```python
from build123d import *

# Parameters (mm, degrees)
EXTRUDE_1_DEPTH              = 3
HOLE_WIZARD_M3_1_D           = 3.4
HOLE_WIZARD_M3_1_DEPTH       = 15
HOLE_WIZARD_M3_1_CSINK_D     = 6.3
HOLE_WIZARD_M3_1_CSINK_ANGLE = 90
HOLE_WIZARD_M3_1_TIP         = 1.021463052


with BuildPart() as part:
    # 草圖1 → 填料-伸長1 (new body)
    with BuildSketch(Plane.XY):
        Polygon((-57.5, -55), (57.5, -55), (57.5, 55), (47.5, 55), (47.5, 95), (-47.5, 95), (-47.5, 55), (-57.5, 55), align=None)
    extrude(amount=EXTRUDE_1_DEPTH)

    # M3 錐坑平頭螺釘的錐孔1
    with Locations(Plane.XY.offset(3)):
        with Locations((-52.5, -50), (-42.5, 90), (-42.5, 50), (42.5, 90), (42.5, 50), (52.5, -50)):
            CounterSinkHole(HOLE_WIZARD_M3_1_D / 2, HOLE_WIZARD_M3_1_CSINK_D / 2, depth=HOLE_WIZARD_M3_1_DEPTH, counter_sink_angle=HOLE_WIZARD_M3_1_CSINK_ANGLE)
            with Locations((0, 0, -(HOLE_WIZARD_M3_1_DEPTH + HOLE_WIZARD_M3_1_TIP / 2))):  # 118° drill point
                Cone(0, HOLE_WIZARD_M3_1_D / 2, HOLE_WIZARD_M3_1_TIP, mode=Mode.SUBTRACT)


solid = part.part
```
Geometry check sheet. Reference: the model listing, model coordinates, mm. A direction names the side the tool comes from. Round coordinates to 2 decimals unless told otherwise and drop trailing zeros. Write each loop counter-clockwise with the first axis right and the second up, starting at its lowest first coordinate (ties: lowest second). Pieces come first, ordered by that corner, then holes. Notation, with made-up numbers: (88, 44) -> (97, 44) arc R30 ccw to (97, 76) -> close; hole circle Ø7 at (20.5, 8.25). An arc over 180 degrees is marked (long way). Put each result on its own line as item: value.
1) Cross-section at C-C, the plane z = 2.3. Enter the section's corners in (x, y).
Recorded:
outline: (-57.5, -55) -> (57.5, -55) -> (57.5, 55) -> (47.5, 55) -> (47.5, 95) -> (-47.5, 95) -> (-47.5, 55) -> (-57.5, 55) -> close; hole circle Ø4.9 at (-52.5, -50); hole circle Ø4.9 at (-42.5, 50); hole circle Ø4.9 at (-42.5, 90); hole circle Ø4.9 at (42.5, 50); hole circle Ø4.9 at (42.5, 90); hole circle Ø4.9 at (52.5, -50)
2) Thickness scan on probe 1 along Y at (x, z) = (-42.5, 0.65); probe 2 along X at (y, z) = (-50, 0.95); probe 3 along Y at (x, z) = (52.5, 1). Record the ranges inside material, lowest first. Write a range as from..to.
Recorded:
probe 1: y = -55..48.3, 51.7..88.3, 91.7..95
probe 2: x = -57.5..-54.2, -50.8..50.8, 54.2..57.5
probe 3: y = -55..-51.7, -48.3..55
3) Cross-section at B-B, the plane x = -42.5. Enter the section's corners in (y, z).
Recorded:
outline: (-55, 0) -> (48.3, 0) -> (48.3, 1.55) -> (46.85, 3) -> (-55, 3) -> close; (51.7, 0) -> (88.3, 0) -> (88.3, 1.55) -> (86.85, 3) -> (53.15, 3) -> (51.7, 1.55) -> close; (91.7, 0) -> (95, 0) -> (95, 3) -> (93.15, 3) -> (91.7, 1.55) -> close
4) Release check for a two-part mould opening along Y. For faces 4 (the face through (57.5, -1, 1)), 5 (the face through (-42.13, 88.34, 0.76)), 6 (the face through (1, 95, 1)) record: pulls with the +Y half, pulls with the -Y half, needs draft (parallel to the pull), parting line crosses it, or undercut.
Recorded:
face 4: needs draft
face 5: undercut
face 6: pulls with the +Y half
5) Depth check by flat-ended pin: P1, Ø0.9, axis at x = -54.5, z = 1, coming from the +Y side; P2, Ø5.5, axis at x = -42.5, y = 90, coming from the +Z side; P3, Ø4.5, axis at x = 42.5, y = 90, coming from the +Z side. Enter the tip coordinate at first touch or a pass-through.
Recorded:
P1: stops at y = 55
P2: stops at z = 2.6
P3: stops at z = 2.1
6) Access from +Z, -Z, +X, -X, +Y, -Y to the whole of each face (thin tool, end or side, straight path). Record for faces 1 (the face through (47.5, 75, 1)), 2 (the face through (-47.5, 75, 1)), 3 (the face through (-1, 21, 3)).
Recorded:
face 1: +Z, -Z, +X, +Y
face 2: +Z, -Z, -X, +Y
face 3: +Z, +X, -X, +Y, -Y
7) Cross-section at D-D, the plane y = 66. Enter the section's corners in (x, z).
Recorded:
outline: (-47.5, 0) -> (47.5, 0) -> (47.5, 3) -> (-47.5, 3) -> close
8) Cross-section at A-A, the plane y = -50. Enter the section's corners in (x, z), plus the area to 3 significant figures.
Recorded:
outline: (-57.5, 0) -> (-54.2, 0) -> (-54.2, 1.55) -> (-55.65, 3) -> (-57.5, 3) -> close; (-50.8, 0) -> (50.8, 0) -> (50.8, 1.55) -> (49.35, 3) -> (-49.35, 3) -> (-50.8, 1.55) -> close; (54.2, 0) -> (57.5, 0) -> (57.5, 3) -> (55.65, 3) -> (54.2, 1.55) -> close
area: 320 mm2
